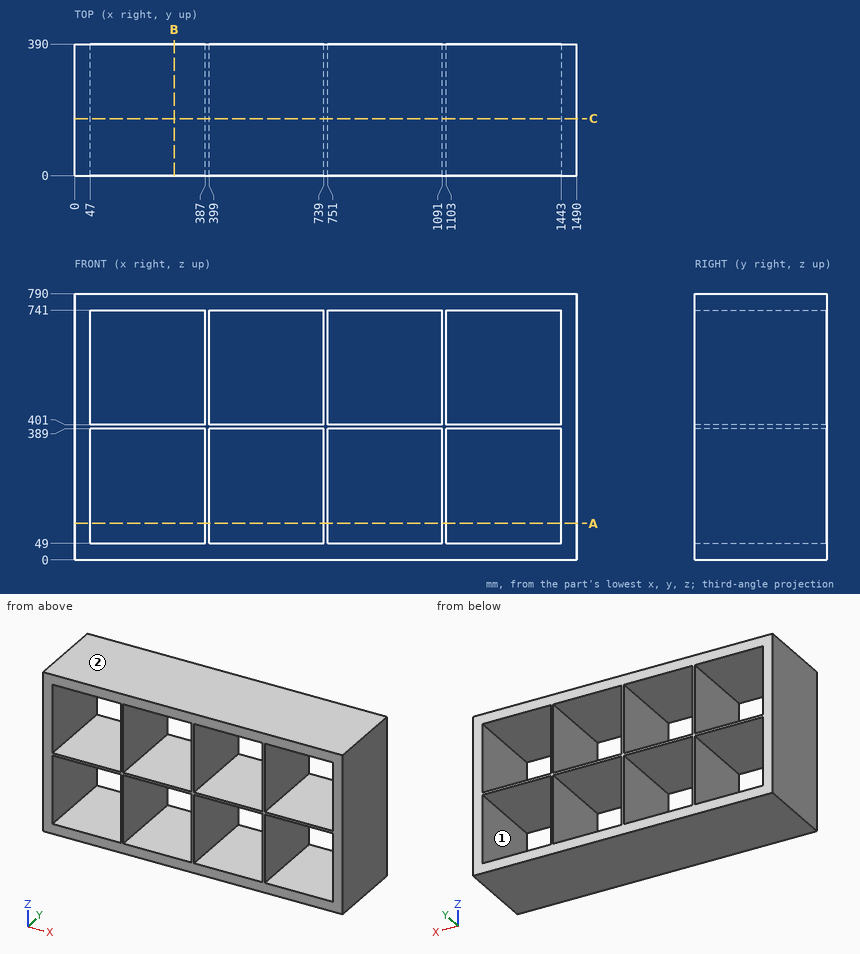
Input: dimensioned drawing with shaded views. Units: mm. Origin: part minimum x, y, z. Coordinates: 2 decimals unless noted, no trailing zeros. Loops run counter-clockwise (first coordinate to the right, second up) from the corner with the lowest first, then second, coordinate; pieces in that order, holes last. Notation, with made-up numbers: (-18.75, 34.25) - (1.25, 34.25) arc R22 ccw to (1.25, 64.25) - close; hole circle Ø8 at (22.25, 81.5). An arc over 180 degrees is marked (long way). One line per question, with ' | ' between items. Start each with the question number.
(1) Ray query, L1, parallel to Z at x = 1394, y = 244.5; L2, parallel to X at y = 115, z = 594. Return the intervals inside material, ascending. Write a range as from..to.
(2) Draft query along Z for the marked faces 1 and 2. Return one class per face: +Z half, -Z half, draft (parallel to the pull), parting line (faces both ways), or undercut.
(3) Cut plane C-C on y = 168.5. Count the separate pieces of the cut face and the enclosed holes in it, and give its area (3 significant figures).
(4) Cut plane A-A on z = 108.5. Output: boundary loops of the cut face in (x, y).
(5) Cut plane B-B on x = 295.5. Output: boundary loops of the cut face in (y, z).
Here are the results:
1) L1: 0..49, 389..401, 741..790 | L2: 0..47, 387..399, 739..751, 1091..1103, 1443..1490
2) face 1: undercut | face 2: +Z half
3) separate pieces: 1 | enclosed holes: 8 | area: 252,000 mm²
4) outline: (0, 0) - (47, 0) - (47, 390) - (0, 390) - close; (387, 0) - (399, 0) - (399, 390) - (387, 390) - close; (739, 0) - (751, 0) - (751, 390) - (739, 390) - close; (1091, 0) - (1103, 0) - (1103, 390) - (1091, 390) - close; (1443, 0) - (1490, 0) - (1490, 390) - (1443, 390) - close
5) outline: (0, 0) - (390, 0) - (390, 49) - (0, 49) - close; (0, 389) - (390, 389) - (390, 401) - (0, 401) - close; (0, 741) - (390, 741) - (390, 790) - (0, 790) - close
